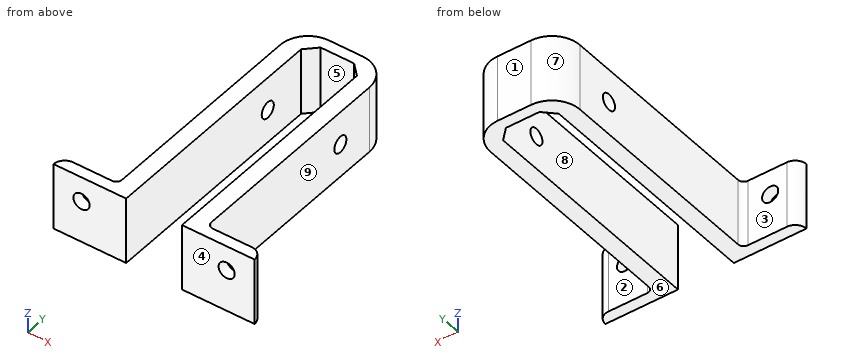
```python
from build123d import *

# Parameters (mm, degrees)
EXTRUDE_1_DEPTH          = 12
CUT_EXTRUDE_1_DEPTH      = 15
CUT_EXTRUDE_1_DEPTH_BACK = 15
SKETCH_2_R               = 1.45
SKETCH_3_R               = 1.45
CUT_EXTRUDE_2_DEPTH      = 15
FILLET_1_R               = 1
FILLET_2_R               = 5
FILLET_3_R               = 2
CHAMFER_1_SIZE           = 2


with BuildPart() as part:
    # 草图1 → 凸台-拉伸1 (new body)
    with BuildSketch(Plane.XY):
        Polygon((0, 0), (13, 0), (13, 44), (23, 44), (23, 0), (36, 0), (36, 2), (26, 2), (26, 46), (10, 46), (10, 2), (0, 2), align=None)
    extrude(amount=EXTRUDE_1_DEPTH)

    # 草图2 → 切除-拉伸1 (cut, two sides: drawn at the far end of the back side and taken through both)
    with BuildSketch(Plane(origin=(13, 0, 0), x_dir=(0, 0, -1), z_dir=(1, 0, 0)).offset(-CUT_EXTRUDE_1_DEPTH_BACK)):
        with Locations(Location((-6, 34, 0), (0, 0, 180))):
            Circle(SKETCH_2_R)
    extrude(amount=CUT_EXTRUDE_1_DEPTH + CUT_EXTRUDE_1_DEPTH_BACK, mode=Mode.SUBTRACT)

    # 草图3 → 切除-拉伸2 (cut)
    with BuildSketch(Plane(origin=(0, 2, 0), x_dir=(1, 0, 0), z_dir=(0, 1, 0))):
        with Locations(Location((5, -7.519173445, 0), (0, 0, 180))):
            Circle(SKETCH_3_R)
        with Locations(Location((31, -7.519173445, 0), (0, 0, 180))):
            Circle(SKETCH_3_R)
    extrude(amount=-CUT_EXTRUDE_2_DEPTH, mode=Mode.SUBTRACT)

    # 圆角1
    fillet_1_edges = [part.edges().sort_by_distance(p)[0] for p in [
        (10, 2, 6),
        (26, 2, 6),
    ]]
    fillet(fillet_1_edges, radius=FILLET_1_R)

    # 圆角2
    fillet_2_edges = [part.edges().sort_by_distance(p)[0] for p in [
        (10, 46, 6),
        (26, 46, 6),
    ]]
    fillet(fillet_2_edges, radius=FILLET_2_R)

    # 圆角3
    fillet_3_edges = [part.edges().sort_by_distance(p)[0] for p in [
        (36, 2, 6),
        (0, 2, 6),
    ]]
    fillet(fillet_3_edges, radius=FILLET_3_R - 0.0001)  # a hair under: the kernel refuses the full size

    # 倒角1
    chamfer_1_edges = [part.edges().sort_by_distance(p)[0] for p in [
        (23, 44, 6),
        (13, 44, 6),
    ]]
    chamfer(chamfer_1_edges, length=CHAMFER_1_SIZE)


solid = part.part
```
CAD build for the part. Positions are in the model's coordinates, mm. Face numbers are marked on the shaded views. A direction names the side the tool comes from. Coordinates: 2 decimals unless noted, no trailing zeros. Write each loop counter-clockwise with the first axis right and the second up, starting at its lowest first coordinate (ties: lowest second). Pieces come first, ordered by that corner, then holes.
(1) Flat gauge pins, fed straight in: pin 1 (3.5 mm diameter, centred on x = 29, z = 5.5, fed in from +Y); pin 2 (2.5 mm diameter, centred on y = 34, z = 6, fed in from -X); pin 3 (4 mm diameter, centred on x = 10.5, z = 10.5, fed in from +Y); pin 4 (6 mm diameter, centred on y = 29, z = 3.5, fed in from +X). Where does each tip first touch, or does it go through?
(2) Cut at C-C, the plane y = 34. List the corners of the cut face in (x, z), and give its area (3 significant figures).
(3) 3-axis set-ups, long thin cutter, end or side, ignore diameter. For the marked faces 1, 2, 3, 4 and 5: which of +Z, -Z, +X, -X, +Y, -Y reach the whole face in a straight line?
(4) Drill centre lines: probe 1 along Y at (x, z) = (11, 6); probe 2 along X at (y, z) = (7, 9); probe 3 along Z at (x, y) = (31, 1.2). Where is each one in solid material? Low to high.
(5) Cut at A-A, the plane x = 31. List the corners of the cut face in (y, z).
(6) Cut at D-D, the plane x = 25. List the corners of the cut face in (y, z).
(7) Two-plate mould, pull along X, no slides. Class the marked faces 6, 7, 8 and 9: +X half, -X half, draft (parallel to the pull), parting line (faces both ways), or undercut.
(8) Cut at B-B, the plane y = 5. List the corners of the cut face in (x, z).
Geometry says:
1. pin 1: stops at y = 2
1. pin 2: passes through
1. pin 3: stops at y = 45.33
1. pin 4: stops at x = 26
2. outline: (10, 0) - (13, 0) - (13, 4.55) - (10, 4.55) - close; (10, 7.45) - (13, 7.45) - (13, 12) - (10, 12) - close; (23, 0) - (26, 0) - (26, 4.55) - (23, 4.55) - close; (23, 7.45) - (26, 7.45) - (26, 12) - (23, 12) - close
2. area: 54.6 mm2
3. face 1: +Z, -Z, +X, -X, +Y
3. face 2: +Z, -Z, +X, +Y
3. face 3: +Z, -Z, -X, +Y
3. face 4: +Z, -Z, +X, -X, -Y
3. face 5: +Z, -Z, -Y
4. probe 1: y = 0 to 32.55, 35.45 to 44
4. probe 2: x = 10 to 13, 23 to 26
4. probe 3: z = 0 to 6.07, 8.97 to 12
5. outline: (0, 0) - (2, 0) - (2, 6.07) - (0, 6.07) - close; (0, 8.97) - (2, 8.97) - (2, 12) - (0, 12) - close
6. outline: (0, 0) - (44, 0) - (44, 12) - (0, 12) - close; hole circle Ø2.9 at (34, 6)
7. face 6: draft
7. face 7: -X half
7. face 8: undercut
7. face 9: +X half
8. outline: (10, 0) - (13, 0) - (13, 12) - (10, 12) - close; (23, 0) - (26, 0) - (26, 12) - (23, 12) - close
